Source: CAD feature listing. Evaluate the final solid. Frame: model axes, mm. Give positions to 0.01 mm unless a question says otherwise; leave off trailing zeros. Order: outer loops, then holes, each group sorted by start corner. A loop starts at its lowest first (then second) coordinate and runs counter-clockwise, first axis right, second up. Notation, with made-up numbers: (-6, -10.5) -> (14, -10.5) arc R25 cw to (14, 16.5) -> close; hole circle Ø10 at (17.5, 29). An arc over 180 degrees is marked (long way). Answer in a Markdown table with one row per item.
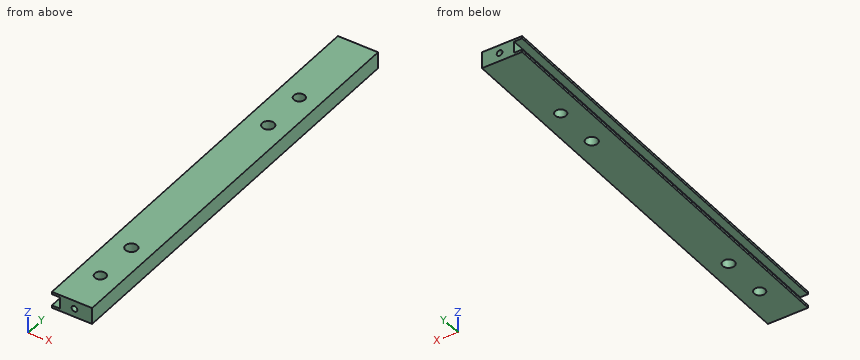
```python
from build123d import *

# Parameters (mm, degrees)
F0_W     = 23.114
F0_H     = 244.602
F1_DEPTH = 9.525
F2_W     = 244.602
F2_H     = 6.6802
F3_DEPTH = 4.572
F4_R     = 3.175
F5_DEPTH = 9.526
F8_D     = 3.3
F8_DEPTH = 10.16
F8_TIP   = 0.9914200214
F9_D     = 3.3
F9_DEPTH = 10.16
F9_TIP   = 0.9914200214
F11_D    = 6.8


with BuildPart() as f1:
    # F0 (on Top) → F1 (new body)
    with BuildSketch(Plane.XY):
        with Locations((-11.557, 122.301)):
            Rectangle(F0_W, F0_H)
    extrude(amount=F1_DEPTH)

    # F2 (on face) → F3 (cut)
    with BuildSketch(Plane(origin=(-23.114, 0, 0), x_dir=(0, -1, 0), z_dir=(-1, 0, 0))):
        with Locations((-122.301, 4.7625)):
            Rectangle(F2_W, F2_H)
    extrude(amount=-F3_DEPTH, mode=Mode.SUBTRACT)

    # F4 (on face) → F5 (cut, through all)
    with BuildSketch(Plane.XY.offset(9.525)):
        with Locations((-11.176, 23.622)):
            Circle(F4_R)
        with Locations((-11.176, 193.8274)):
            Circle(F4_R)
    extrude(amount=-F5_DEPTH, mode=Mode.SUBTRACT)

    # F8
    with Locations(Plane(origin=(0, 244.602, 0), x_dir=(-1, 0, 0), z_dir=(0, 1, 0))):
        with Locations((10.16, 4.7752)):
            Hole(F8_D / 2, depth=F8_DEPTH)
            with Locations((0, 0, -(F8_DEPTH + F8_TIP / 2))):  # 118° drill point
                Cone(0, F8_D / 2, F8_TIP, mode=Mode.SUBTRACT)

    # F9
    with Locations(Plane.XZ):
        with Locations((-10.16, 4.7752)):
            Hole(F9_D / 2, depth=F9_DEPTH)
            with Locations((0, 0, -(F9_DEPTH + F9_TIP / 2))):  # 118° drill point
                Cone(0, F9_D / 2, F9_TIP, mode=Mode.SUBTRACT)

    # F11 (through all)
    with Locations(Plane.XY.offset(9.525)):
        with Locations((-11.176, 167.2717), (-11.176, 50.1777)):
            Hole(F11_D / 2)


solid = f1.part
```
(1) Ray query, probe 1 along Y at (x, z) = (-11.25, 1.75); probe 2 along X at (y, z) = (24, 7.25); probe 3 along Y at (x, z) = (-9.5, 9.25). Return the intervals inside material, ascending.
A:
| item | result |
|---|---|
| probe 1 | y = 0 to 20.45, 26.8 to 46.78, 53.58 to 163.87, 170.67 to 190.65, 197 to 244.6 |
| probe 2 | x = -18.54 to -14.33, -8.02 to 0 |
| probe 3 | y = 0 to 20.93, 26.32 to 47.22, 53.14 to 164.31, 170.23 to 191.13, 196.52 to 244.6 |
(2) First-contact query: pin 1 Ø6 at (x, y) = (-11.18, 167.27) entering from +Z; pin 2 Ø3 at (x, z) = (-10.16, 4.78) entering from +Y. Flat tips, straight axial feed; report the tip coordinate or a pass-through.
A:
| item | result |
|---|---|
| pin 1 | passes through |
| pin 2 | stops at y = 234.35 |
(3) Section query A-A (y = 60). Return the cut outline in (x, z) (3 decimals), plus the area to 3 significant figures.
A:
| item | result |
|---|---|
| outline | (-23.114, 0) -> (0, 0) -> (0, 9.525) -> (-23.114, 9.525) -> (-23.114, 8.103) -> (-18.542, 8.103) -> (-18.542, 1.422) -> (-23.114, 1.422) -> close |
| area | 190 mm^2 |
